```python
from build123d import *

# Parameters (mm, degrees)
CROQUIS2_R              = 3.38
SALIENTE_EXTRUIR1_DEPTH = 3
CROQUIS4_W              = 19
CROQUIS4_H              = 3
SALIENTE_EXTRUIR2_DEPTH = 10
REDONDEO1_R             = 10
CROQUIS7_W              = 2
CROQUIS7_H              = 4
SALIENTE_EXTRUIR4_DEPTH = 10
REDONDEO4_R             = 1.5
REDONDEO5_R             = 2
REDONDEO6_R             = 3


# Some blends are built 0.0001 mm under size
with BuildPart() as part:
    # Croquis2 → Saliente-Extruir1 (new body)
    with BuildSketch(Plane.XY):
        with BuildLine():
            Line((-9.5, 0), (-9.5, -29))
            Line((-9.5, -29), (9.5, -29))
            Line((9.5, -29), (9.5, 0))
            ThreePointArc((9.5, 0), (0, 9.5), (-9.5, 0))
        make_face()
        Circle(CROQUIS2_R, mode=Mode.SUBTRACT)
    extrude(amount=SALIENTE_EXTRUIR1_DEPTH)

    # Croquis4 → Saliente-Extruir2 (add)
    with BuildSketch(Plane.XY.offset(3)):
        with Locations((0, -27.5)):
            Rectangle(CROQUIS4_W, CROQUIS4_H)
    extrude(amount=SALIENTE_EXTRUIR2_DEPTH)

    # Redondeo1
    redondeo1_edges = [part.edges().sort_by_distance(p)[0] for p in [
        (0, -26, 3),
    ]]
    fillet(redondeo1_edges, radius=REDONDEO1_R - 0.0001)  # a hair under: the kernel refuses the full size

    # Croquis7 → Saliente-Extruir4 (add)
    with BuildSketch(Plane.XY.offset(3)):
        with Locations((-8.5, -8.38)):
            Rectangle(CROQUIS7_W, CROQUIS7_H)
        with Locations((8.5, -8.38)):
            Rectangle(CROQUIS7_W, CROQUIS7_H)
    extrude(amount=SALIENTE_EXTRUIR4_DEPTH)

    # Redondeo4
    redondeo4_edges = [part.edges().sort_by_distance(p)[0] for p in [
        (-8.5, -6.38, 3),
        (-8.5, -10.38, 3),
        (8.5, -6.38, 3),
        (8.5, -10.38, 3),
    ]]
    fillet(redondeo4_edges, radius=REDONDEO4_R)

    # Redondeo5
    redondeo5_edges = [part.edges().sort_by_distance(p)[0] for p in [
        (8.5, -10.38, 13),
        (8.5, -6.38, 13),
        (-8.5, -10.38, 13),
        (-8.5, -6.38, 13),
    ]]
    fillet(redondeo5_edges, radius=REDONDEO5_R - 0.0001)  # a hair under: the kernel refuses the full size

    # Redondeo6
    # the kernel refuses this fillet: 3 mm, written as the material it takes off along each edge
    with BuildSketch(Plane(origin=(16.122828959, -26, 13), x_dir=(0, -1, 0), z_dir=(-1, 0, 0))) as redondeo6_piece_1:
        with BuildLine():
            CenterArc((2.649131583, -3), REDONDEO6_R, 90, 76.657984638)
            Line((-0.269898159, -2.307710059), (-0.561801133, -2.238481065))
            ThreePointArc((-0.561801133, -2.238481065), (-0.3, -0.0001), (-0.3, 0))
            Line((-0.3, 0), (0, 0.3))
            Line((0, 0.3), (2.649131583, 0.3))
            Line((2.649131583, 0.3), (2.649131583, 0))
        make_face()
    extrude(amount=32.245657917, mode=Mode.SUBTRACT)


solid = part.part
```
Design review of the part built by this model. Coordinates are the model's own, in mm. A direction names the side the tool comes from. Coordinates: 2 decimals unless noted, no trailing zeros. Write each loop counter-clockwise with the first axis right and the second up, starting at its lowest first coordinate (ties: lowest second). Pieces come first, ordered by that corner, then holes.
1) Add section C-C (y = -11). Write out the cut boundary in (x, z), plus the area to 3 significant figures.
2) Add section B-B (z = 6.75). Write out the cut boundary in (x, y).
3) Add section A-A (x = 0). Write out the cut boundary in (y, z).
4) Mouldability with a two-part tool opening along X and no side actions: class faces 1 (the flat face through (-9.5, -18, 2)), 2 (the flat face through (0, -6, 3)), 3 (the cylindrical face through (8.5, -5.9, 3.4)) as +X half, -X half, draft (parallel to the pull), parting line (faces both ways), or undercut.
5) To check wall thickness, follow L1, parallel to Y at x = 0, z = 2.35; L2, parallel to Z at x = 7.25, y = -9; L3, parallel to X at y = -9, z = 10.25. State the ranges of each line that lie inside material, in increasing order.
6) Add section D-D (z = 2). Write out the cut boundary in (x, y).
7) Insertion check: pin 1 (5 mm diameter, centred on x = -2.5, z = 10.5, fed in from +Y); pin 2 (9.5 mm diameter, centred on x = 4, y = 0.5, fed in from +Z); pin 3 (6 mm diameter, centred on x = 3, y = -15, fed in from +Z). Each pin has a flat end and moves straight along its axis. Give the tip position at first contact, or say it passes through.
8) Machinability: for faces 4 (the flat face through (8, -6.38, 8)), 5 (the cylindrical face through (-8.49, -10.83, 3.43)), 6 (the cylindrical face through (3.224, 1.015, 1.479)), which of the approach directions +Z, -Z, +X, -X, +Y, -Y give a long, thin tool a straight path to every point of the face, cutting with its end or side? Answer none if there is none.
Check result:
1. outline: (-9.5, 0) - (9.5, 0) - (9.5, 3.29) - (7.5, 3.29) - (7.5, 3) - (-7.5, 3) - (-7.5, 3.29) - (-9.5, 3.29) - close
1. area: 58.1 mm2
2. outline: (-9.5, -29) - (9.5, -29) - (9.5, -23.81) - (-9.5, -23.81) - close; (-9.5, -10.38) - (-7.5, -10.38) - (-7.5, -6.38) - (-9.5, -6.38) - close; (7.5, -10.38) - (9.5, -10.38) - (9.5, -6.38) - (7.5, -6.38) - close
3. outline: (-29, 0) - (-3.38, 0) - (-3.38, 3) - (-16, 3) arc R10 cw to (-25.73, 10.69) arc R3 ccw to (-28.65, 13) - (-29, 13) - close; (3.38, 0) - (9.5, 0) - (9.5, 3) - (3.38, 3) - close
4. face 1: -X half
4. face 2: undercut
4. face 3: draft
5. L1: y = -29 to -3.38, 3.38 to 9.5
5. L2: z = 0 to 3
5. L3: x = -9.5 to -7.5, 7.5 to 9.5
6. outline: (-9.5, -29) - (9.5, -29) - (9.5, 0) arc R9.5 ccw to (-9.5, 0) - close; hole circle Ø6.76 at (0, 0)
7. pin 1: stops at y = -24.66
7. pin 2: stops at z = 3
7. pin 3: stops at z = 3.2
8. face 4: +Z, +X, -X, +Y
8. face 5: +Z, +X, -X
8. face 6: +Z, -Z
